Autodesk Inventor part; units mm, degrees
ref_plane "YZ Plane" through (0, 0, 0) normal (1, 0, 0) x (0, 1, 0)
ref_plane "XZ Plane" through (0, 0, 0) normal (0, 1, 0) x (-1, 0, 0)
ref_plane "XY Plane" through (0, 0, 0) normal (0, 0, 1) x (1, 0, 0)
sketch "Sketch1" plane through (0, 0, 0) normal (0, 0, 1) x (1, 0, 0)
  circle A0 centre (0, 0) radius 16
  circle A1 centre (0, 0) radius 5
  dimension "d0" = 32
  dimension "d1" = 10
extrude "Extrusion1" add sketch "Sketch1" along normal mid plane 8
sketch "Sketch2" plane through (0, 0, 4) normal (0, 0, 1) x (1, 0, 0)
  circle A0 centre (0, 0) radius 5
  arc A1 (-1.483, -4.775) -> (1.483, -4.775) centre (0, -5) ccw
  arc A2 (1.483, 4.775) -> (-1.483, 4.775) centre (0, 5) ccw
  dimension "d4" = 3
  dimension "d5" = 3
extrude "Extrusion2" cut sketch "Sketch2" against normal blind 8 contours A0 A2 | A1 A0
sketch "Sketch3" plane through (0, 0, 4) normal (0, 0, 1) x (1, 0, 0)
  point P0 (0, 0)
  point P1 (-12, 0)
  dimension "d8" = 12
hole "Hole1" at (-12, 0, 4) direction (0, 0, -1) diameter 4.134 depth 8
fillet "Fillet1" radius 0.75 1 edges at (-16, 0, 4)
properties part number "45"
Verification items for the finished model (mm, model axes). A direction names the side the tool comes from. Give positions to 0.01 mm unless a question says otherwise; leave off trailing zeros. Write each loop counter-clockwise with the first axis right and the second up, starting at its lowest first coordinate (ties: lowest second). Pieces come first, ordered by that corner, then holes. Notation, with made-up numbers: (12.25, -1) - (50.25, -1) arc R16 cw to (50.25, 13) - close; hole circle Ø9 at (-14, 2). An arc over 180 degrees is marked (long way). Answer as CSV lines item,"result". Start each with the question number.
1. Sectioned sample at A-A (x = 0). Record the boundary of the cut face in (y, z).
2. Set-up check for faces 1 (the face through (-5, 0, 0)), 2 (the face through (-4, 4, -4)): record each of +Z, -Z, +X, -X, +Y, -Y from which the full face is reachable in a straight line by a thin tool's end or side.
3. Sectioned sample at B-B (y = 0). Record the boundary of the cut face in (x, z), then the cut area to 3 significant figures.
4. Sectioned sample at C-C (z = 0.5). Record the boundary of the cut face in (x, y) (3 decimals), then the cut area to 3 significant figures.
5. Thickness scan on line 1 (Y direction, x = 0, z = -1); line 2 (X direction, y = 0.5, z = 2); line 3 (Y direction, x = -10.5, z = -2.75). Record the ranges inside material, lowest first.
6. Draft check along X on faces 3 (the face through (-3.47, 15.62, -0.43)), 4 (the face through (-9.982, 0.448, -0.056)), 5 (the face through (-4, 4, 4)). Enter one of: pulls with the +X half, pulls with the -X half, needs draft (parallel to the pull), parting line crosses it, or undercut.
7. Depth check by flat-ended pin: pin 1 (1.5 mm diameter, centred on y = -1, z = -2.5, fed in from +X); pin 2 (1 mm diameter, centred on x = -3.5, z = 1, fed in from +Y); pin 3 (4 mm diameter, centred on x = -4, z = 2, fed in from +Y); pin 4 (1.8 mm diameter, centred on x = 0, y = 5, fed in from -Z). Enter the tip coordinate at first touch or a pass-through.
Derived:
1,outline,"(-16, -4) - (-6.5, -4) - (-6.5, 4) - (-15.25, 4) arc R0.75 ccw to (-16, 3.25) - close; (6.5, -4) - (16, -4) - (16, 3.25) arc R0.75 ccw to (15.25, 4) - (6.5, 4) - close"
2,face 1,"+Z, -Z"
2,face 2,"-Z, +X, -X, +Y, -Y"
3,outline,"(-16, -4) - (-14.07, -4) - (-14.07, 4) - (-15.25, 4) arc R0.75 ccw to (-16, 3.25) - close; (-9.93, -4) - (-5, -4) - (-5, 4) - (-9.93, 4) - close; (5, -4) - (16, -4) - (16, 3.25) arc R0.75 ccw to (15.25, 4) - (5, 4) - close"
3,area,"143 mm²"
4,outline,"circle Ø32 at (0, 0); hole circle Ø4.134 at (-12, 0); hole (-1.483, -4.775) arc R1.5 ccw (long way) to (1.483, -4.775) arc R5 ccw to (1.483, 4.775) arc R1.5 ccw (long way) to (-1.483, 4.775) arc R5 ccw to start"
4,area,"705 mm²"
5,line 1,"-16 to -6.5, 6.5 to 16"
5,line 2,"-15.99 to -14.01, -9.99 to -4.97, 4.97 to 15.99"
5,line 3,"-12.07 to -1.42, 1.42 to 12.07"
6,face 3,"parting line crosses it"
6,face 4,"undercut"
6,face 5,"needs draft"
7,pin 1,"x = 16"
7,pin 2,"y = 15.72"
7,pin 3,"y = 15.87"
7,pin 4,"through"
